Design review of the part built by this model. Coordinates are the model's own, in mm. Face numbers are marked on the shaded views. A direction names the side the tool comes from. Give positions to 0.01 mm unless a question says otherwise; leave off trailing zeros. Loops run counter-clockwise (first coordinate to the right, second up) from the corner with the lowest first, then second, coordinate; pieces in that order, holes last. Notation, with made-up numbers: M -26.75,85 L 12.25,85 A25 cw 12.25,108 Z; hole C 11,34 d10. An arc over 180 degrees is marked long. Use a Markdown table: item, result. Add a question column.
(1) For probe 1 along Y at (x, z) = (14, 1.05); probe 2 along Y at (x, z) = (14.08, 0.9); probe 3 along X at (y, z) = (-31, 2.1), list the stretches that pass through material, from the lowest coordinate up.
(2) For the marked faces 1 and 2, list the 3-axis set-ups (+Z, -Z, +X, -X, +Y, -Y) from which the entire face can be reached by the end or side of a thin tool; tool diameter is ignored.
(3) Add section C-C, the plane z = 0.95. Give the boundary of the cut face in (x, y), then the cut area to 3 significant figures.
(4) Insertion check: pin 1 Ø1.5 at (y, z) = (5, 3) entering from -X; pin 2 Ø21 at (x, y) = (-3.5, 0.5) entering from +Z; pin 3 Ø9 at (x, y) = (-14.08, -26.49) entering from +Z; pin 4 Ø2 at (y, z) = (-14, 3) entering from +X. Each pin has a flat end and moves straight along its axis. Give the tip position at first contact, or say it passes through.
(5) Add section A-A, the plane y = 0. Give the boundary of the cut face in (x, z), then the cut area to 4 significant figures.
(6) Add section D-D, the plane y = 26.49. Give the boundary of the cut face in (x, z), then the cut area to 3 significant figures.
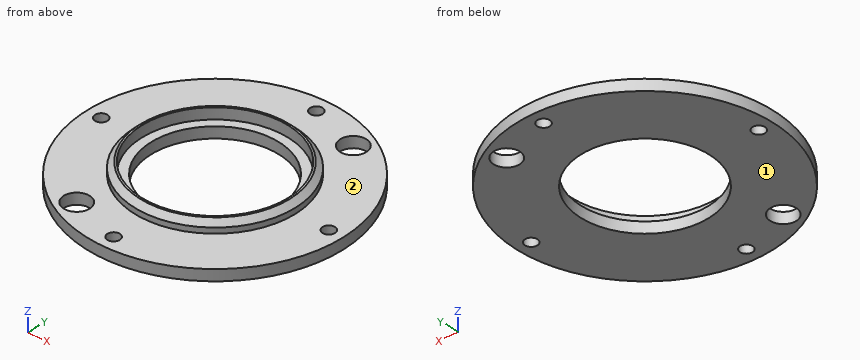
```python
from build123d import *

# Parameters (mm, degrees)
SKIZZE1_R                        = 35
SKIZZE1_R_2                      = 17.5
AUFSATZ_LINEAR_AUSTRAGEN1_DEPTH  = 3
SKIZZE2_R                        = 22
SKIZZE2_R_2                      = 20
AUFSATZ_LINEAR_AUSTRAGEN2_DEPTH  = 3
FASE1_SIZE                       = 1.5
KREISMUSTER2_COUNT               = 4
F_7_1_7_1_DURCHMESSER_BOHRUNG1_D = 7.1
KREISMUSTER3_COUNT               = 2


with BuildPart() as part:
    # Skizze1 → Aufsatz-Linear austragen1 (new body)
    with BuildSketch(Plane.XY):
        Circle(SKIZZE1_R)
        Circle(SKIZZE1_R_2, mode=Mode.SUBTRACT)
    extrude(amount=AUFSATZ_LINEAR_AUSTRAGEN1_DEPTH)

    # Skizze2 → Aufsatz-Linear austragen2 (add)
    with BuildSketch(Plane.XY.offset(3)):
        Circle(SKIZZE2_R)
        Circle(SKIZZE2_R_2, mode=Mode.SUBTRACT)
    extrude(amount=AUFSATZ_LINEAR_AUSTRAGEN2_DEPTH)

    # Fase1
    fase1_edges = [part.edges().sort_by_distance(p)[0] for p in [
        (-22, 0, 6),
    ]]
    chamfer(fase1_edges, length=FASE1_SIZE)

    # Skizze4 → 3.4 _3.4_ Durchmesser Bohrung1 (revolve, cut)
    with BuildSketch(Plane(origin=(0, 31, 0), x_dir=(0, 1, 0), z_dir=(1, 0, 0))):
        Polygon((0, 0), (0, 11.021463052), (1.7, 10), (1.7, 0), align=None)
    f_3_4_3_4_durchmesser_bohrung1 = revolve(axis=Axis((0, 31, -6.35), (0, 0, 1)), mode=Mode.SUBTRACT)

    # Kreismuster2: 3.4 _3.4_ Durchmesser Bohrung1 ×4 about axis
    kreismuster2_axis = Axis((0, 0, 0), (0, 0, 1))
    for i in range(1, KREISMUSTER2_COUNT):
        add(f_3_4_3_4_durchmesser_bohrung1.rotate(kreismuster2_axis, i * 360 / KREISMUSTER2_COUNT), mode=Mode.SUBTRACT)

    # 7.1 _7.1_ Durchmesser Bohrung1 (through all)
    with Locations(Plane(origin=(0, 0, 0), x_dir=(-1, 0, 0), z_dir=(0, 0, -1))):
        with Locations((-14.08, 26.49)):
            f_7_1_7_1_durchmesser_bohrung1 = Hole(F_7_1_7_1_DURCHMESSER_BOHRUNG1_D / 2)

    # Kreismuster3: 7.1 _7.1_ Durchmesser Bohrung1 ×2 about axis
    kreismuster3_axis = Axis((0, 0, 0), (0, 0, 1))
    for i in range(1, KREISMUSTER3_COUNT):
        add(f_7_1_7_1_durchmesser_bohrung1.rotate(kreismuster3_axis, i * 360 / KREISMUSTER3_COUNT), mode=Mode.SUBTRACT)


solid = part.part
```
Established:
| question | item | result |
|---|---|---|
| 1 | probe 1 | -32.08 to -10.5, 10.5 to 22.94, 30.04 to 32.08 |
| 1 | probe 2 | -32.04 to -10.39, 10.39 to 22.94, 30.04 to 32.04 |
| 1 | probe 3 | -16.25 to -1.7, 1.7 to 16.25 |
| 2 | face 1 | -Z, +X, -X, +Y, -Y |
| 2 | face 2 | +Z |
| 3 | outline | C 0,0 d70; hole C -31,0 d3.4; hole C -14.08,-26.49 d7.1; hole C 0,0 d35; hole C 0,-31 d3.4; hole C 0,31 d3.4; hole C 14.08,26.49 d7.1; hole C 31,0 d3.4 |
| 3 | area | 2,770 mm^2 |
| 4 | pin 1 | x = -34.74 |
| 4 | pin 2 | through |
| 4 | pin 3 | z = 3 |
| 4 | pin 4 | x = 32.5 |
| 5 | outline | M -35,0 L -32.7,0 L -32.7,3 L -35,3 Z; M -29.3,0 L -17.5,0 L -17.5,3 L -20,3 L -20,6 L -20.5,6 L -22,4.5 L -22,3 L -29.3,3 Z; M 17.5,0 L 29.3,0 L 29.3,3 L 22,3 L 22,4.5 L 20.5,6 L 20,6 L 20,3 L 17.5,3 Z; M 32.7,0 L 35,0 L 35,3 L 32.7,3 Z |
| 5 | area | 94.35 mm^2 |
| 6 | outline | M -22.88,0 L 10.53,0 L 10.53,3 L -22.88,3 Z; M 17.63,0 L 22.88,0 L 22.88,3 L 17.63,3 Z |
| 6 | area | 116 mm^2 |
